from build123d import *

# Parameters (mm, degrees)
SKETCH1_W            = 50.8
SKETCH1_H            = 50.8
BOSS_EXTRUDE1_DEPTH  = 5.461
CUT_EXTRUDE1_DEPTH   = 5.461
M5_CLEARANCE_HOLE1_D = 5.5


with BuildPart() as part:
    # Sketch1 → Boss-Extrude1 (new body)
    with BuildSketch(Plane(origin=(0, 0, 0), x_dir=(1, 0, 0), z_dir=(0, 1, 0))):
        with Locations((25.4, 25.4)):
            Rectangle(SKETCH1_W, SKETCH1_H)
    extrude(amount=BOSS_EXTRUDE1_DEPTH)

    # Sketch2 → Cut-Extrude1 (cut)
    with BuildSketch(Plane(origin=(0, 5.461, 0), x_dir=(1, 0, 0), z_dir=(0, 1, 0))):
        Polygon((28.1305, 28.1305), (39.327666667, 28.1305), (39.327666667, 22.6695), (28.1305, 22.6695), (28.1305, 11.472333333), (22.6695, 11.472333333), (22.6695, 22.6695), (11.472333333, 22.6695), (11.472333333, 28.1305), (22.6695, 28.1305), (22.6695, 39.327666667), (28.1305, 39.327666667), align=None)
    extrude(amount=-CUT_EXTRUDE1_DEPTH, mode=Mode.SUBTRACT)

    # M5 Clearance Hole1 (through all)
    with Locations(Plane(origin=(0, 5.461, 0), x_dir=(1, 0, 0), z_dir=(0, 1, 0))):
        with Locations((7.62, 43.18), (43.18, 43.18), (43.18, 7.62), (7.62, 7.62)):
            Hole(M5_CLEARANCE_HOLE1_D / 2)


solid = part.part
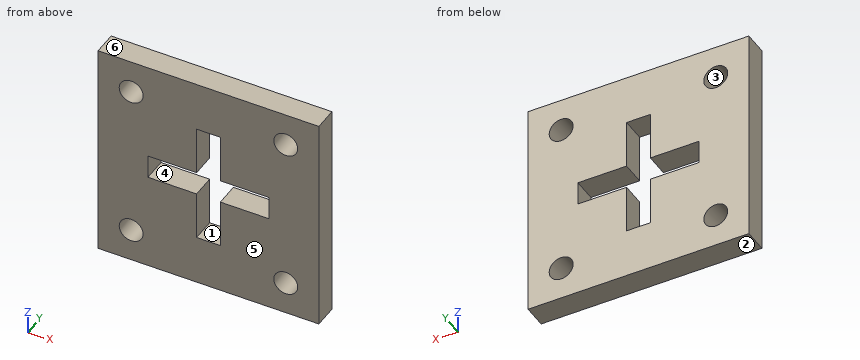
Could you check a few things on this model? Use its own coordinates, in mm. Face numbers are marked on the shaded views. A direction names the side the tool comes from. Round coordinates to 2 decimals unless told otherwise and drop trailing zeros. Order: outer loops, then holes, each group sorted by start corner. A loop starts at its lowest first (then second) coordinate and runs counter-clockwise, first axis right, second up.
Q1. Thinking about a two-plate mould opening in Z: for the marked faces 3, 4, 5 and 6, which applies, released by +Z, released by -Z, zero draft, split by the parting line, or undercut?
Geometry says:
face 3: undercut
face 4: undercut
face 5: zero draft
face 6: released by +Z
Q2. Imagine slicing it at D-D, the plane x = 43.18. List the corners of the cut face in (y, z) for me, then the cut area to 3 significant figures.
Geometry says:
outline: (0, -50.8) - (5.46, -50.8) - (5.46, -45.93) - (0, -45.93) - close; (0, -40.43) - (5.46, -40.43) - (5.46, -10.37) - (0, -10.37) - close; (0, -4.87) - (5.46, -4.87) - (5.46, 0) - (0, 0) - close
area: 217 mm2
Q3. Imagine slicing it at A-A, the plane x = 18.5. List the corners of the cut face in (y, z) for me.
Geometry says:
outline: (0, -50.8) - (5.46, -50.8) - (5.46, -28.13) - (0, -28.13) - close; (0, -22.67) - (5.46, -22.67) - (5.46, 0) - (0, 0) - close
Q4. Which directions (+Z, -Z, +X, -X, +Y, -Y) give clear straight access to the entire face, cutting with the end or side of a thin tool? Please do the marked faces 1 and 2.
Geometry says:
face 1: +Y, -Y
face 2: -Z, +X, -X, +Y, -Y
Q5. Please list where these lines run through material, in increasing order: probe 1 along Z at (x, y) = (7.62, 2); probe 2 along X at (y, z) = (3.4, -43.18); probe 3 along X at (y, z) = (1.45, -34).
Geometry says:
probe 1: z = -50.8 to -45.93, -40.43 to -10.37, -4.87 to 0
probe 2: x = 0 to 4.87, 10.37 to 40.43, 45.93 to 50.8
probe 3: x = 0 to 22.67, 28.13 to 50.8
Q6. Imagine slicing it at C-C, the plane y = 2.35. List the corners of the cut face in (x, z) for me.
Geometry says:
outline: (0, -50.8) - (50.8, -50.8) - (50.8, 0) - (0, 0) - close; hole circle Ø5.5 at (7.62, -43.18); hole circle Ø5.5 at (7.62, -7.62); hole (11.47, -28.13) - (22.67, -28.13) - (22.67, -39.33) - (28.13, -39.33) - (28.13, -28.13) - (39.33, -28.13) - (39.33, -22.67) - (28.13, -22.67) - (28.13, -11.47) - (22.67, -11.47) - (22.67, -22.67) - (11.47, -22.67) - close; hole circle Ø5.5 at (43.18, -43.18); hole circle Ø5.5 at (43.18, -7.62)
Q7. Imagine slicing it at B-B, the plane z = -7.62. List the corners of the cut face in (x, y) for me.
Geometry says:
outline: (0, 0) - (4.87, 0) - (4.87, 5.46) - (0, 5.46) - close; (10.37, 0) - (40.43, 0) - (40.43, 5.46) - (10.37, 5.46) - close; (45.93, 0) - (50.8, 0) - (50.8, 5.46) - (45.93, 5.46) - close
